from build123d import *

# Parameters (mm, degrees)
SKETCH1_W               = 190.5
SKETCH1_H               = 107.95
BOSS_EXTRUDE1_DEPTH     = 6.35
SKETCH2_W               = 12.7
SKETCH2_H               = 6.35
CUT_EXTRUDE1_DEPTH      = 7.35
LPATTERN1_COUNT         = 8
LPATTERN1_PITCH         = 25.4
MIRROR1_COPY_1_SKETCH_W = 12.7
MIRROR1_COPY_1_SKETCH_H = 6.35
MIRROR1_COPY_1_DEPTH    = 7.35
MIRROR1_COPY_2_SKETCH_W = 12.7
MIRROR1_COPY_2_SKETCH_H = 6.35
MIRROR1_COPY_2_DEPTH    = 7.35
MIRROR1_COPY_3_SKETCH_W = 12.7
MIRROR1_COPY_3_SKETCH_H = 6.35
MIRROR1_COPY_3_DEPTH    = 7.35
MIRROR1_COPY_4_SKETCH_W = 12.7
MIRROR1_COPY_4_SKETCH_H = 6.35
MIRROR1_COPY_4_DEPTH    = 7.35
MIRROR1_COPY_5_SKETCH_W = 12.7
MIRROR1_COPY_5_SKETCH_H = 6.35
MIRROR1_COPY_5_DEPTH    = 7.35
MIRROR1_COPY_6_SKETCH_W = 12.7
MIRROR1_COPY_6_SKETCH_H = 6.35
MIRROR1_COPY_6_DEPTH    = 7.35
MIRROR1_COPY_7_SKETCH_W = 12.7
MIRROR1_COPY_7_SKETCH_H = 6.35
MIRROR1_COPY_7_DEPTH    = 7.35
SKETCH3_W               = 6.35
SKETCH3_H               = 12.7
CUT_EXTRUDE2_DEPTH      = 7.35
LPATTERN2_COUNT         = 3
LPATTERN2_PITCH         = 25.4
MIRROR2_COPY_1_SKETCH_W = 6.35
MIRROR2_COPY_1_SKETCH_H = 12.7
MIRROR2_COPY_1_DEPTH    = 7.35
MIRROR2_COPY_2_SKETCH_W = 6.35
MIRROR2_COPY_2_SKETCH_H = 12.7
MIRROR2_COPY_2_DEPTH    = 7.35
SKETCH4_W               = 25.4
SKETCH4_H               = 4.7625
CUT_EXTRUDE3_DEPTH      = 7.35
SKETCH5_W               = 73.025
SKETCH5_H               = 25.4
CUT_EXTRUDE4_DEPTH      = 7.35
SKETCH6_W               = 50.8
SKETCH6_H               = 25.4
CUT_EXTRUDE5_DEPTH      = 7.35


with BuildPart() as part:
    # Sketch1 → Boss-Extrude1 (new body)
    with BuildSketch(Plane.XY):
        Rectangle(SKETCH1_W, SKETCH1_H)
    extrude(amount=BOSS_EXTRUDE1_DEPTH)

    # Sketch2 → Cut-Extrude1 (cut, through all)
    with BuildSketch(Plane.XY.offset(6.35)):
        with Locations((-88.9, -50.8)):
            Rectangle(SKETCH2_W, SKETCH2_H)
    cut_extrude1 = extrude(amount=-CUT_EXTRUDE1_DEPTH, mode=Mode.SUBTRACT)

    # LPattern1: Cut-Extrude1 ×8
    with Locations(*[(i * LPATTERN1_PITCH, 0, 0) for i in range(1, LPATTERN1_COUNT)]):
        add(cut_extrude1, mode=Mode.SUBTRACT)

    # Mirror1: Cut-Extrude1 across plane
    add(cut_extrude1.mirror(Plane.ZX), mode=Mode.SUBTRACT)

    # Mirror1 copy 1 sketch → Mirror1 copy 1 (cut, through all)
    with BuildSketch(Plane(origin=(25.4, 0, 6.35), x_dir=(1, 0, 0), z_dir=(0, 0, 1))):
        with Locations((-88.9, 50.8)):
            Rectangle(MIRROR1_COPY_1_SKETCH_W, MIRROR1_COPY_1_SKETCH_H)
    extrude(amount=-MIRROR1_COPY_1_DEPTH, mode=Mode.SUBTRACT)

    # Mirror1 copy 2 sketch → Mirror1 copy 2 (cut, through all)
    with BuildSketch(Plane(origin=(50.8, 0, 6.35), x_dir=(1, 0, 0), z_dir=(0, 0, 1))):
        with Locations((-88.9, 50.8)):
            Rectangle(MIRROR1_COPY_2_SKETCH_W, MIRROR1_COPY_2_SKETCH_H)
    extrude(amount=-MIRROR1_COPY_2_DEPTH, mode=Mode.SUBTRACT)

    # Mirror1 copy 3 sketch → Mirror1 copy 3 (cut, through all)
    with BuildSketch(Plane(origin=(76.2, 0, 6.35), x_dir=(1, 0, 0), z_dir=(0, 0, 1))):
        with Locations((-88.9, 50.8)):
            Rectangle(MIRROR1_COPY_3_SKETCH_W, MIRROR1_COPY_3_SKETCH_H)
    extrude(amount=-MIRROR1_COPY_3_DEPTH, mode=Mode.SUBTRACT)

    # Mirror1 copy 4 sketch → Mirror1 copy 4 (cut, through all)
    with BuildSketch(Plane(origin=(101.6, 0, 6.35), x_dir=(1, 0, 0), z_dir=(0, 0, 1))):
        with Locations((-88.9, 50.8)):
            Rectangle(MIRROR1_COPY_4_SKETCH_W, MIRROR1_COPY_4_SKETCH_H)
    extrude(amount=-MIRROR1_COPY_4_DEPTH, mode=Mode.SUBTRACT)

    # Mirror1 copy 5 sketch → Mirror1 copy 5 (cut, through all)
    with BuildSketch(Plane(origin=(127, 0, 6.35), x_dir=(1, 0, 0), z_dir=(0, 0, 1))):
        with Locations((-88.9, 50.8)):
            Rectangle(MIRROR1_COPY_5_SKETCH_W, MIRROR1_COPY_5_SKETCH_H)
    extrude(amount=-MIRROR1_COPY_5_DEPTH, mode=Mode.SUBTRACT)

    # Mirror1 copy 6 sketch → Mirror1 copy 6 (cut, through all)
    with BuildSketch(Plane(origin=(152.4, 0, 6.35), x_dir=(1, 0, 0), z_dir=(0, 0, 1))):
        with Locations((-88.9, 50.8)):
            Rectangle(MIRROR1_COPY_6_SKETCH_W, MIRROR1_COPY_6_SKETCH_H)
    extrude(amount=-MIRROR1_COPY_6_DEPTH, mode=Mode.SUBTRACT)

    # Mirror1 copy 7 sketch → Mirror1 copy 7 (cut, through all)
    with BuildSketch(Plane(origin=(177.8, 0, 6.35), x_dir=(1, 0, 0), z_dir=(0, 0, 1))):
        with Locations((-88.9, 50.8)):
            Rectangle(MIRROR1_COPY_7_SKETCH_W, MIRROR1_COPY_7_SKETCH_H)
    extrude(amount=-MIRROR1_COPY_7_DEPTH, mode=Mode.SUBTRACT)

    # Sketch3 → Cut-Extrude2 (cut, through all)
    with BuildSketch(Plane.XY.offset(6.35)):
        with Locations((-92.075, 28.575)):
            Rectangle(SKETCH3_W, SKETCH3_H)
    cut_extrude2 = extrude(amount=-CUT_EXTRUDE2_DEPTH, mode=Mode.SUBTRACT)

    # LPattern2: Cut-Extrude2 ×3
    with Locations(*[(0, -i * LPATTERN2_PITCH, 0) for i in range(1, LPATTERN2_COUNT)]):
        add(cut_extrude2, mode=Mode.SUBTRACT)

    # Mirror2: Cut-Extrude2 across plane
    add(cut_extrude2.mirror(Plane(origin=(0, 0, 0), x_dir=(0, 0, 1), z_dir=(1, 0, 0))), mode=Mode.SUBTRACT)

    # Mirror2 copy 1 sketch → Mirror2 copy 1 (cut, through all)
    with BuildSketch(Plane(origin=(0, -25.4, 6.35), x_dir=(-1, 0, 0), z_dir=(0, 0, 1))):
        with Locations((-92.075, -28.575)):
            Rectangle(MIRROR2_COPY_1_SKETCH_W, MIRROR2_COPY_1_SKETCH_H)
    extrude(amount=-MIRROR2_COPY_1_DEPTH, mode=Mode.SUBTRACT)

    # Mirror2 copy 2 sketch → Mirror2 copy 2 (cut, through all)
    with BuildSketch(Plane(origin=(0, -50.8, 6.35), x_dir=(-1, 0, 0), z_dir=(0, 0, 1))):
        with Locations((-92.075, -28.575)):
            Rectangle(MIRROR2_COPY_2_SKETCH_W, MIRROR2_COPY_2_SKETCH_H)
    extrude(amount=-MIRROR2_COPY_2_DEPTH, mode=Mode.SUBTRACT)

    # Sketch4 → Cut-Extrude3 (cut, through all)
    with BuildSketch(Plane.XY.offset(6.35)):
        with Locations((-38.1, 30.00375)):
            Rectangle(SKETCH4_W, SKETCH4_H)
    extrude(amount=-CUT_EXTRUDE3_DEPTH, mode=Mode.SUBTRACT)

    # Sketch5 → Cut-Extrude4 (cut, through all)
    with BuildSketch(Plane.XY.offset(6.35)):
        with Locations((39.6875, -15.875)):
            Rectangle(SKETCH5_W, SKETCH5_H)
    extrude(amount=-CUT_EXTRUDE4_DEPTH, mode=Mode.SUBTRACT)

    # Sketch6 → Cut-Extrude5 (cut, through all)
    with BuildSketch(Plane.XY.offset(6.35)):
        with Locations((38.1, 22.225)):
            Rectangle(SKETCH6_W, SKETCH6_H)
    extrude(amount=-CUT_EXTRUDE5_DEPTH, mode=Mode.SUBTRACT)


solid = part.part
Verification items for the finished model (mm, model axes). A direction names the side the tool comes from. Coordinates: 2 decimals unless noted, no trailing zeros. Loops run counter-clockwise (first coordinate to the right, second up) from the corner with the lowest first, then second, coordinate; pieces in that order, holes last. Notation, with made-up numbers: M 18.25,36.5 L 44.25,36.5 A11 ccw 44.25,42.5 Z; hole C -7,47.5 d5. An arc over 180 degrees is marked long. One line per item, written item: value.
1. Gauge pin test, flat ends, axial feed: P1, Ø1.9, axis at x = -93.5, z = 3.5, coming from the -Y side (3 decimals); P2, Ø1.9, axis at y = 50.5, z = 3, coming from the -X side; P3, Ø3, axis at y = -51.5, z = 3.5, coming from the +X side. Record the tip position at first contact, or that the pin passes through.
Answers follow:
P1: y = -47.625
P2: x = -82.55
P3: x = 82.55
2. Section check D-D on z = 5. Give the number of separate pieces and of enclosed holes in the cut face, plus the area to 3 significant figures.
Answers follow:
separate pieces: 1
enclosed holes: 3
area: 15,500 mm^2
3. Section check A-A on x = 37.5. Record the cut outline in (y, z) (3 decimals).
Answers follow:
outline: M -47.625,0 L -28.575,0 L -28.575,6.35 L -47.625,6.35 Z; M -3.175,0 L 9.525,0 L 9.525,6.35 L -3.175,6.35 Z; M 34.925,0 L 47.625,0 L 47.625,6.35 L 34.925,6.35 Z
4. Material ranges on line 1 along Y through (x, z) = (26, 5) (3 decimals); line 2 along Y through (x, z) = (13.5, 2.75) (3 decimals); line 3 along X through (y, z) = (-5, 3.25) (3 decimals), recorded low to high. Write a range as from..to.
Answers follow:
line 1: -53.975..-28.575, -3.175..9.525, 34.925..53.975
line 2: -47.625..-28.575, -3.175..9.525, 34.925..47.625
line 3: -95.25..3.175, 76.2..95.25
5. Mould release check, pull along Y, two halves, no side actions. Record for faces 4 (the flat face through (-38, 32.385, 3)), 5 (the flat face through (-25, 53.975, 3)), 6 (the flat face through (82.55, 51, 3)): pulls with the +Y half, pulls with the -Y half, needs draft (parallel to the pull), parting line crosses it, or undercut.
Answers follow:
face 4: undercut
face 5: pulls with the +Y half
face 6: needs draft
6. Section check B-B on y = -26.5. Record the cut outline in (x, z) (3 decimals).
Answers follow:
outline: M -88.9,0 L 3.175,0 L 3.175,6.35 L -88.9,6.35 Z; M 76.2,0 L 88.9,0 L 88.9,6.35 L 76.2,6.35 Z
7. Set-up check for faces 1 (the flat face through (44.45, 51, 3)), 2 (the flat face through (-92, 22.225, 3)), 3 (the flat face through (-13, -47.625, 3)): record each of +Z, -Z, +X, -X, +Y, -Y from which the full face is reachable in a straight line by a thin tool's end or side.
Answers follow:
face 1: +Z, -Z, +Y
face 2: +Z, -Z, -X
face 3: +Z, -Z, -Y
